Part model, mm, in its own coordinate system. Face numbers are marked on the shaded views. A direction names the side the tool comes from. Give positions to 0.01 mm unless a question says otherwise; leave off trailing zeros. Write each loop counter-clockwise with the first axis right and the second up, starting at its lowest first coordinate (ties: lowest second). Pieces come first, ordered by that corner, then holes.
from build123d import *

# Parameters (mm, degrees)
F1_DEPTH = 63.5
F0_W     = 18.70497
F0_H     = 19.05
F2_DEPTH = 25.4
F3_DEPTH = 7.9375
F0_W_2   = 25.4
F0_H_2   = 28.575
F5_R     = 5.08


with BuildPart() as f1:
    # F0 (on Front) → F1 (new body, symmetric)
    with BuildSketch(Plane.XZ):
        Polygon((-41.275, 9.525), (-41.275, -9.525), (41.275, -9.525), (41.275, 9.525), (22.225, 9.525), align=None)
    extrude(amount=F1_DEPTH, both=True)

    # F0 (on Front) → F2 (join, symmetric)
    with BuildSketch(Plane.XZ):
        with BuildLine():
            Line((22.225, 9.525), (41.275, 9.525))
            Line((41.275, 9.525), (41.275, 27.0002))
            ThreePointArc((41.275, 27.0002), (45.92468, 38.22552), (57.15, 42.8752))
            Line((57.15, 42.8752), (60.325, 42.8752))
            Line((60.325, 42.8752), (60.325, 61.9252))
            Line((60.325, 61.9252), (57.15, 61.9252))
            add(Edge.make_bspline(
                [(56.126842, 61.91021), (56.468024, 61.915997), (56.809083, 61.920993), (57.15, 61.9252)],
                knots=[110.703053, 110.703053, 110.703053, 110.703053, 111.504536, 111.504536, 111.504536, 111.504536], degree=3))
            ThreePointArc((56.126842, 61.91021), (32.095166, 51.331475), (22.225, 27.0002))
            Line((22.225, 27.0002), (22.225, 9.525))
        make_face()
        with Locations((69.677485, 52.4002)):
            Rectangle(F0_W, F0_H)
    extrude(amount=F2_DEPTH, both=True)

    # F0 (on Front) → F3 (join, symmetric)
    with BuildSketch(Plane.XZ):
        with BuildLine():
            add(Edge.make_bspline(
                [(-41.275, 9.525), (-40.465312, 45.22587), (9.001882, 61.110903), (56.126842, 61.91021)],
                knots=[0, 0, 0, 0, 110.703053, 110.703053, 110.703053, 110.703053], degree=3))
            Line((-41.275, 9.525), (22.225, 9.525))
            Line((22.225, 9.525), (22.225, 27.0002))
            ThreePointArc((22.225, 27.0002), (32.095166, 51.331475), (56.126842, 61.91021))
        make_face()
    extrude(amount=F3_DEPTH, both=True)

    # F0 (on Front) → F4 (revolve)
    with BuildSketch(Plane.XZ):
        with Locations((98.425, 52.3875)):
            Rectangle(F0_W_2, F0_H_2)
    revolve(axis=Axis((85.725, 0, 52.3875), (0, 0, -1)))

    # F5
    f5_edges = [f1.edges().sort_by_distance(p)[0] for p in [
        (41.275, -63.5, 0),
        (-41.275, -63.5, 0),
        (41.275, 63.5, 0),
        (-41.275, 63.5, 0),
    ]]
    fillet(f5_edges, radius=F5_R)


solid = f1.part
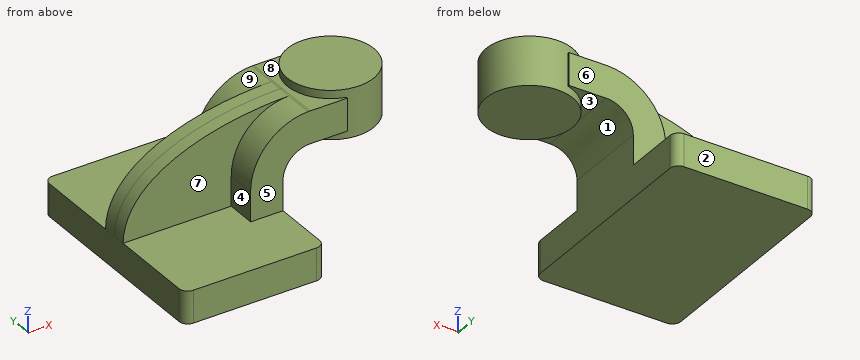
1) Mould opens along X. For the marked faces 1, 2, 3 and 4 say: +X half, -X half, draft (parallel to the pull), parting line (faces both ways), or undercut.
Check result:
face 1: undercut
face 2: draft
face 3: undercut
face 4: -X half
2) Flat gauge pins, fed straight in: P1, Ø14, axis at y = 17, z = 15, coming from the -X side (3 decimals); P2, Ø11, axis at x = 72.5, y = -12, coming from the -Z side; P3, Ø4, axis at x = 1, y = 39.5, coming from the +Z side (3 decimals); P4, Ø2, axis at x = 31.5, z = 58.5, coming from the +Y side. Where does each tip first touch, or does it go through?
Check result:
P1: stops at x = -41.275
P2: stops at z = 38.1
P3: stops at z = 9.525
P4: stops at y = 7.94
3) Drill centre lines: L1, parallel to Z at x = 39, y = 48.5 (3 decimals); L2, parallel to Y at x = 32, z = 53; L3, parallel to Y at x = 42, z = 46.5. Where is each one in solid material? Low to high.
Check result:
L1: z = -9.525 to 9.525
L2: y = -7.94 to 7.94
L3: y = -25.4 to 25.4
4) 3-axis set-ups, long thin cutter, end or side, ignore diameter. For the marked faces 5, 6, 7, 8 and 9: which of +Z, -Z, +X, -X, +Y, -Y reach the whole face in a straight line?
Check result:
face 5: +Z, +X, -X, -Y
face 6: +Z, +X, -X, +Y
face 7: +Z, -X, -Y
face 8: +Z, -X
face 9: +Z, -X, +Y
5) Saw through at B-B (x = 96). Write the cut outline in (y, z) (3 decimals), and give its area (3 significant figures).
Check result:
outline: (-23.229, 38.1) - (23.229, 38.1) - (23.229, 66.675) - (-23.229, 66.675) - close
area: 1,330 mm2
6) Saw through at A-A (z = -0.5). Write the cut outline in (x, y) (3 decimals).
Check result:
outline: (-41.275, -58.42) arc R5.08 ccw to (-36.195, -63.5) - (36.195, -63.5) arc R5.08 ccw to (41.275, -58.42) - (41.275, 58.42) arc R5.08 ccw to (36.195, 63.5) - (-36.195, 63.5) arc R5.08 ccw to (-41.275, 58.42) - close
7) Saw through at C-C (y = 33.5). Write the cut outline in (x, z) (3 decimals).
Check result:
outline: (-41.275, -9.525) - (41.275, -9.525) - (41.275, 9.525) - (-41.275, 9.525) - close
